from build123d import *

# Parameters (mm, degrees)
SKETCH1_W           = 42
SKETCH1_H           = 42
SKETCH1_R           = 1.5
BOSS_EXTRUDE1_DEPTH = 33
CHAMFER1_SIZE       = 4
SKETCH2_R           = 11
BOSS_EXTRUDE2_DEPTH = 2
SKETCH3_R           = 2.5
BOSS_EXTRUDE3_DEPTH = 22


with BuildPart() as part:
    # Sketch1 → Boss-Extrude1 (new body)
    with BuildSketch(Plane(origin=(0, 0, 0), x_dir=(1, 0, 0), z_dir=(0, 1, 0))):
        Rectangle(SKETCH1_W, SKETCH1_H)
        with Locations(Location((15.5, 15.5, 0), (0, 0, 270))):
            Circle(SKETCH1_R, mode=Mode.SUBTRACT)
        with Locations(Location((-15.5, 15.5, 0), (0, 0, 270))):
            Circle(SKETCH1_R, mode=Mode.SUBTRACT)
        with Locations(Location((15.5, -15.5, 0), (0, 0, 90))):
            Circle(SKETCH1_R, mode=Mode.SUBTRACT)
        with Locations(Location((-15.5, -15.5, 0), (0, 0, 90))):
            Circle(SKETCH1_R, mode=Mode.SUBTRACT)
    extrude(amount=BOSS_EXTRUDE1_DEPTH)

    # Chamfer1
    chamfer1_edges = [part.edges().sort_by_distance(p)[0] for p in [
        (21, 16.5, 21),
        (-21, 16.5, 21),
        (-21, 16.5, -21),
        (21, 16.5, -21),
    ]]
    chamfer(chamfer1_edges, length=CHAMFER1_SIZE)

    # Sketch2 → Boss-Extrude2 (add)
    with BuildSketch(Plane(origin=(0, 33, 0), x_dir=(1, 0, 0), z_dir=(0, 1, 0))):
        with Locations(Location((0, 0, 0), (0, 0, 270))):
            Circle(SKETCH2_R)
    extrude(amount=BOSS_EXTRUDE2_DEPTH)

    # Sketch3 → Boss-Extrude3 (add)
    with BuildSketch(Plane(origin=(0, 35, 0), x_dir=(1, 0, 0), z_dir=(0, 1, 0))):
        with Locations(Location((0, 0, 0), (0, 0, 270))):
            Circle(SKETCH3_R)
    extrude(amount=BOSS_EXTRUDE3_DEPTH)


solid = part.part
The model under review builds one solid part; all positions refer to its coordinate system, in mm. A direction names the side the tool comes from. Coordinates: 2 decimals unless noted, no trailing zeros. Loops run counter-clockwise (first coordinate to the right, second up) from the corner with the lowest first, then second, coordinate; pieces in that order, holes last.
(1) Insertion check: P1, Ø2, axis at x = -8.5, z = -11.5, coming from the +Y side. The pin has a flat end and moves straight along its axis. Give the tip position at first contact, or say it passes through.
Determined:
P1: stops at y = 33
(2) Tool access review of faces 4 (the cylindrical face through (15.57, 16.27, -17)), 5 (the cylindrical face through (-10.74, 33.99, -2.38)): name each direction out of +Z, -Z, +X, -X, +Y, -Y from which nothing blocks a thin tool from reaching the whole face with its end or side.
Determined:
face 4: +Y, -Y
face 5: +Y
(3) Consider section A-A, the plane z = -15.5. Give the boundary of the cut face in (x, y).
Determined:
outline: (-21, 0) - (-17, 0) - (-17, 33) - (-21, 33) - close; (-14, 0) - (14, 0) - (14, 33) - (-14, 33) - close; (17, 0) - (21, 0) - (21, 33) - (17, 33) - close
(4) Wall thickness on L1, parallel to X at y = 22, z = 15.5; L2, parallel to X at y = 14, z = -15: over which ranges is each line inside the solid? List them lowest first.
Determined:
L1: x = -21 to -17, -14 to 14, 17 to 21
L2: x = -21 to -16.91, -14.09 to 14.09, 16.91 to 21
(5) Consider section B-B, the plane x = -15.5. Give the boundary of the cut face in (y, z), plus the area to 3 significant figures.
Determined:
outline: (0, -21) - (33, -21) - (33, -17) - (0, -17) - close; (0, -14) - (33, -14) - (33, 14) - (0, 14) - close; (0, 17) - (33, 17) - (33, 21) - (0, 21) - close
area: 1,190 mm2
(6) Draft analysis for pull direction Z (two halves, no side actions). For faces 1 (the flat face through (0, 16, 21)), 2 (the flat face through (0, 57, 0)), 3 (the cylindrical face through (-15.43, 16.27, -17)), state which applies: +Z half, -Z half, draft (parallel to the pull), parting line (faces both ways), or undercut.
Determined:
face 1: +Z half
face 2: draft
face 3: undercut
(7) Consider section D-D, the plane x = 0. Give the boundary of the cut face in (y, z).
Determined:
outline: (0, -21) - (33, -21) - (33, -11) - (35, -11) - (35, -2.5) - (57, -2.5) - (57, 2.5) - (35, 2.5) - (35, 11) - (33, 11) - (33, 21) - (0, 21) - close
(8) Consider section C-C, the plane y = 24. Give the boundary of the cut face in (x, z), plus the area to 3 significant figures.
Determined:
outline: (-21, -17) - (-17, -21) - (17, -21) - (21, -17) - (21, 17) - (17, 21) - (-17, 21) - (-21, 17) - close; hole circle Ø3 at (-15.5, -15.5); hole circle Ø3 at (-15.5, 15.5); hole circle Ø3 at (15.5, -15.5); hole circle Ø3 at (15.5, 15.5)
area: 1,700 mm2
